Geometry check sheet. Reference: the model listing, model coordinates, mm. A direction names the side the tool comes from. Give positions to 0.01 mm unless a question says otherwise; leave off trailing zeros. Write each loop counter-clockwise with the first axis right and the second up, starting at its lowest first coordinate (ties: lowest second). Pieces come first, ordered by that corner, then holes. Notation, with made-up numbers: (37.5, 83) -> (86.5, 83) arc R20 ccw to (86.5, 94) -> close; hole circle Ø2 at (-8, 73). An arc over 180 degrees is marked (long way). One line per item, written item: value.
from build123d import *

# Parameters (mm, degrees)
SKETCH1_W               = 105.25
SKETCH1_H               = 26
BOSS_EXTRUDE1_DEPTH     = 13
SKETCH1_3_W             = 10.5
SKETCH1_3_H             = 19.5
BOSS_EXTRUDE2_DEPTH     = 5.25
SKETCH2_R               = 10.25
CUT_EXTRUDE1_DEPTH      = 111.918044069
CUT_EXTRUDE2_REACH      = 72.772
CUT_EXTRUDE2_END_RADIUS = 10.25
SKETCH3_R               = 2.75
FILLET1_R               = 5
FILLET4_R               = 2.75


with BuildPart() as part:
    # Sketch1 → Boss-Extrude1 (new, symmetric)
    with BuildSketch(Plane.XY):
        Rectangle(SKETCH1_W, SKETCH1_H)
    extrude(amount=BOSS_EXTRUDE1_DEPTH, both=True)

    # Sketch1<3> → Boss-Extrude2 (add, symmetric)
    with BuildSketch(Plane.XY):
        with Locations((-7.625, 22.75)):
            Rectangle(SKETCH1_3_W, SKETCH1_3_H)
        with Locations((47.375, 22.75)):
            Rectangle(SKETCH1_3_W, SKETCH1_3_H)
    extrude(amount=BOSS_EXTRUDE2_DEPTH, both=True)

    # Sketch2 → Cut-Extrude1 (cut, through all)
    with BuildSketch(Plane.ZY.offset(52.625)):
        Circle(SKETCH2_R)
    extrude(amount=-CUT_EXTRUDE1_DEPTH, mode=Mode.SUBTRACT)

    # Cut-Extrude2: up to this cylinder (the profile starts outside it)
    cut_extrude2_end = Plane(origin=(19.875, 0, 0), z_dir=(-1, 0, 0)) * Cylinder(CUT_EXTRUDE2_END_RADIUS, 222.044, mode=Mode.PRIVATE)
    # Sketch3 → Cut-Extrude2 (cut, up to the surface)
    with BuildSketch(Plane(origin=(0, 32.5, 0), x_dir=(1, 0, 0), z_dir=(0, 1, 0)), mode=Mode.PRIVATE) as cut_extrude2_sk1:
        with Locations(Location((-7.625, 0, 0), (0, 0, 270))):
            Circle(SKETCH3_R)
    cut_extrude2_tool1 = extrude(cut_extrude2_sk1.sketch, amount=-CUT_EXTRUDE2_REACH, mode=Mode.PRIVATE) - cut_extrude2_end
    add(cut_extrude2_tool1.solids().sort_by_distance((-7.625, 32.5, 0))[0], mode=Mode.SUBTRACT)
    # Sketch3 → Cut-Extrude2 (cut, up to the surface)
    with BuildSketch(Plane(origin=(0, 32.5, 0), x_dir=(1, 0, 0), z_dir=(0, 1, 0)), mode=Mode.PRIVATE) as cut_extrude2_sk2:
        with Locations(Location((47.375, 0, 0), (0, 0, 270))):
            Circle(SKETCH3_R)
    cut_extrude2_tool2 = extrude(cut_extrude2_sk2.sketch, amount=-CUT_EXTRUDE2_REACH, mode=Mode.PRIVATE) - cut_extrude2_end
    add(cut_extrude2_tool2.solids().sort_by_distance((47.375, 32.5, 0))[0], mode=Mode.SUBTRACT)

    # Fillet1
    fillet1_edges = [part.edges().sort_by_distance(p)[0] for p in [
        (0, 13, 13),
        (0, -13, 13),
        (0, -13, -13),
        (0, 13, -13),
    ]]
    fillet(fillet1_edges, radius=FILLET1_R)

    # Fillet4
    fillet4_edges = [part.edges().sort_by_distance(p)[0] for p in [
        (-12.875, 13, 0),
        (42.125, 13, 0),
        (-2.375, 13, 0),
        (47.375, 13, -5.25),
        (47.375, 13, 5.25),
        (-7.625, 13, 5.25),
        (-7.625, 13, -5.25),
    ]]
    fillet(fillet4_edges, radius=FILLET4_R - 0.0001)  # a hair under: the kernel refuses the full size


solid = part.part
1) Mould release check, pull along X, two halves, no side actions. Record for faces 1 (the flat face through (-52.625, -6, 9)), 2 (the flat face through (47, 24, -5.25)), 3 (the flat face through (-2.375, 24, 0)): released by +X, released by -X, zero draft, split by the parting line, or undercut.
Verdict:
face 1: released by -X
face 2: zero draft
face 3: undercut
2) Sectioned sample at B-B on x = 8.5. Record the cut outline in (y, z), plus the area to 3 significant figures.
Verdict:
outline: (-13, -8) arc R5 ccw to (-8, -13) -> (8, -13) arc R5 ccw to (13, -8) -> (13, 8) arc R5 ccw to (8, 13) -> (-8, 13) arc R5 ccw to (-13, 8) -> close; hole circle Ø20.5 at (0, 0)
area: 324 mm^2
3) Sectioned sample at A-A on y = 0. Record the cut outline in (x, z) (3 decimals).
Verdict:
outline: (-52.625, -13) -> (52.625, -13) -> (52.625, -10.25) -> (-52.625, -10.25) -> close; (-52.625, 10.25) -> (52.625, 10.25) -> (52.625, 13) -> (-52.625, 13) -> close
4) Sectioned sample at D-D on z = 9. Record the cut outline in (x, y) (3 decimals).
Verdict:
outline: (-52.625, -12.899) -> (52.625, -12.899) -> (52.625, -4.905) -> (-52.625, -4.905) -> close; (-52.625, 4.905) -> (52.625, 4.905) -> (52.625, 12.899) -> (-52.625, 12.899) -> close
5) Depth check by flat-ended pin: pin 1 Ø5 at (x, y) = (-8, 26) entering from -Z; pin 2 Ø3 at (x, y) = (48.5, 27) entering from +Z; pin 3 Ø8.5 at (y, z) = (28, 2.5) entering from -X (3 decimals). Enter the tip coordinate at first touch or a pass-through.
Verdict:
pin 1: z = -5.25
pin 2: z = 5.25
pin 3: x = -12.875
6) Tool access check on faces 4 (the cylindrical face through (50.1, 21.35, -0.36)), 5 (the cylindrical face through (41.298, 13.784, 0.112)), 6 (the flat face through (-8, 24, -5.25)), 7 (the cylindrical face through (-7.51, 13.78, 6.08)), 8 (the flat face through (45, 32.5, 2)). Record the directions out of +Z, -Z, +X, -X, +Y, -Y that give a thin tool (end or side, any length) a straight path to the whole face; none if there is none.
Verdict:
face 4: +Y
face 5: +Z, -Z, +Y
face 6: -Z, +X, -X, +Y
face 7: +Z, +X, -X, +Y
face 8: +Z, -Z, +X, -X, +Y
7) Sectioned sample at C-C on z = 0. Record the cut outline in (x, y) (3 decimals).
Verdict:
outline: (-52.625, -13) -> (52.625, -13) -> (52.625, -10.25) -> (-52.625, -10.25) -> close; (-52.625, 10.25) -> (-10.375, 10.25) -> (-10.375, 32.5) -> (-12.875, 32.5) -> (-12.875, 15.75) arc R2.75 cw to (-15.625, 13) -> (-52.625, 13) -> close; (-4.875, 10.25) -> (44.625, 10.25) -> (44.625, 32.5) -> (42.125, 32.5) -> (42.125, 15.75) arc R2.75 cw to (39.375, 13) -> (0.375, 13) arc R2.75 cw to (-2.375, 15.75) -> (-2.375, 32.5) -> (-4.875, 32.5) -> close; (50.125, 10.25) -> (52.625, 10.25) -> (52.625, 32.5) -> (50.125, 32.5) -> close
8) Scan lines: probe 1 along X at (y, z) = (22.25, 0) (3 decimals); probe 2 along Z at (x, y) = (-38.5, -0.5); probe 3 along X at (y, z) = (23.5, 1.5) (3 decimals). Record each from-to range of solid material in increasing order.
Verdict:
probe 1: -12.875 to -10.375, -4.875 to -2.375, 42.125 to 44.625, 50.125 to 52.625
probe 2: -13 to -10.24, 10.24 to 13
probe 3: -12.875 to -9.93, -5.32 to -2.375, 42.125 to 45.07, 49.68 to 52.625
